```python
from build123d import *

# Parameters (mm, degrees)
SKETCH_2_W               = 20
SKETCH_2_H               = 30
EXTRUDE_1_DEPTH          = 60
SKETCH_3_W               = 18
SKETCH_3_H               = 28
CUT_EXTRUDE_1_DEPTH      = 61
CUT_EXTRUDE_1_DEPTH_BACK = 61
SKETCH_5_W               = 20
SKETCH_5_H               = 14
CUT_EXTRUDE_3_DEPTH      = 1
CUT_EXTRUDE_3_DEPTH_BACK = 31
SKETCH_6_R               = 2.025
CUT_EXTRUDE_4_DEPTH      = 31
SKETCH_7_R               = 2.025
CUT_EXTRUDE_5_DEPTH      = 1
CUT_EXTRUDE_5_DEPTH_BACK = 31


with BuildPart() as part:
    # 草图2 → 凸台-拉伸1 (new body, symmetric)
    with BuildSketch(Plane(origin=(0, 0, 0), x_dir=(1, 0, 0), z_dir=(0, 1, 0))):
        Rectangle(SKETCH_2_W, SKETCH_2_H)
    extrude(amount=EXTRUDE_1_DEPTH, both=True)

    # 草图3 → 切除-拉伸1 (cut, two sides)
    with BuildSketch(Plane(origin=(0, 0, 0), x_dir=(1, 0, 0), z_dir=(0, 1, 0))) as cut_extrude_1_sk:
        Rectangle(SKETCH_3_W, SKETCH_3_H)
    extrude(amount=CUT_EXTRUDE_1_DEPTH, mode=Mode.SUBTRACT)
    extrude(cut_extrude_1_sk.sketch, amount=-CUT_EXTRUDE_1_DEPTH_BACK, mode=Mode.SUBTRACT)

    # 草图5 → 切除-拉伸3 (cut, two sides)
    with BuildSketch(Plane.XY.offset(15)) as cut_extrude_3_sk:
        with Locations((0, -53)):
            Rectangle(SKETCH_5_W, SKETCH_5_H)
    extrude(amount=CUT_EXTRUDE_3_DEPTH, mode=Mode.SUBTRACT)
    extrude(cut_extrude_3_sk.sketch, amount=-CUT_EXTRUDE_3_DEPTH_BACK, mode=Mode.SUBTRACT)

    # 草图6 → 切除-拉伸4 (cut, through all)
    with BuildSketch(Plane.XY.offset(15)):
        with Locations((0, -33.5)):
            Circle(SKETCH_6_R)
    extrude(amount=-CUT_EXTRUDE_4_DEPTH, mode=Mode.SUBTRACT)

    # 草图7 → 切除-拉伸5 (cut, two sides)
    with BuildSketch(Plane.XY.offset(15)) as cut_extrude_5_sk:
        with Locations((0, 50)):
            Circle(SKETCH_7_R)
        with Locations((0, 30)):
            Circle(SKETCH_7_R)
        with Locations((0, 10)):
            Circle(SKETCH_7_R)
    extrude(amount=CUT_EXTRUDE_5_DEPTH, mode=Mode.SUBTRACT)
    extrude(cut_extrude_5_sk.sketch, amount=-CUT_EXTRUDE_5_DEPTH_BACK, mode=Mode.SUBTRACT)


solid = part.part
```
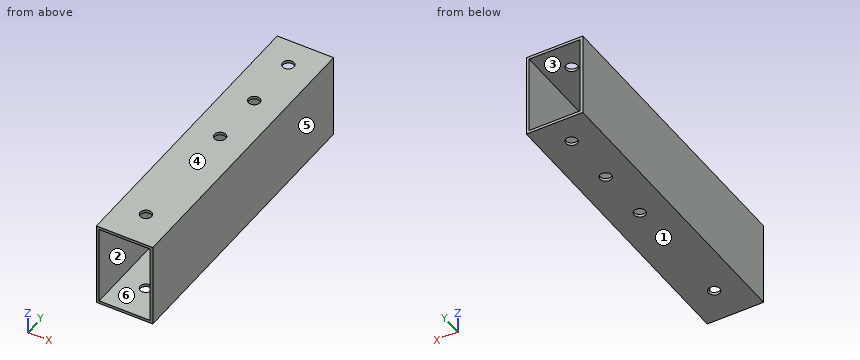
Input: part model. Units: mm. Frame: model coordinates. Face numbers are marked on the shaded views. A direction names the side the tool comes from. Give positions to 0.01 mm unless a question says otherwise; leave off trailing zeros. Order: outer loops, then holes, each group sorted by start corner. A loop starts at its lowest first (then second) coordinate and runs counter-clockwise, first axis right, second up. Notation, with made-up numbers: M -36,17.5 L 15,17.5 A21 ccw 15,33.5 Z; hole C -22,-6 d10. An arc over 180 degrees is marked long. Return JSON: item names as keys, results as strings.
Item 1: Ray query, probe 1 along Y at (x, z) = (0, -14.25) (3 decimals); probe 2 along Z at (x, y) = (-5.25, 18); probe 3 along X at (y, z) = (-36, -4.25). Return the intervals inside material, ascending.
Solutions:
{"probe 1": "-46 to -35.525, -31.475 to 7.975, 12.025 to 27.975, 32.025 to 47.975, 52.025 to 60", "probe 2": "-15 to -14, 14 to 15", "probe 3": "-10 to -9, 9 to 10"}
Item 2: Cut plane A-A (y = 47). Return loops of the section in (x, z).
Solutions:
{"outline": "M -10,-15 L 10,-15 L 10,15 L -10,15 Z; hole M -9,-14 L 9,-14 L 9,14 L -9,14 Z"}
Item 3: Pull-direction query (X, two-part tool) for the marked faces 3, 4, 5 and 6; classes: +X half, -X half, draft (parallel to the pull), parting line (faces both ways), or undercut.
Solutions:
{"face 3": "undercut", "face 4": "draft", "face 5": "+X half", "face 6": "undercut"}
Item 4: Cut plane C-C (z = -7). Return loops of the section in (x, y), then the cut area to 3 significant figures.
Solutions:
{"outline": "M -10,-46 L -9,-46 L -9,60 L -10,60 Z; M 9,-46 L 10,-46 L 10,60 L 9,60 Z", "area": "212 mm^2"}
Item 5: Cut plane B-B (x = 5.25). Return loops of the section in (y, z).
Solutions:
{"outline": "M -46,-15 L 60,-15 L 60,-14 L -46,-14 Z; M -46,14 L 60,14 L 60,15 L -46,15 Z"}
Item 6: Cut plane D-D (y = -33.5). Return loops of the section in (x, z) (3 decimals).
Solutions:
{"outline": "M -10,-15 L -2.025,-15 L -2.025,-14 L -9,-14 L -9,14 L -2.025,14 L -2.025,15 L -10,15 Z; M 2.025,-15 L 10,-15 L 10,15 L 2.025,15 L 2.025,14 L 9,14 L 9,-14 L 2.025,-14 Z"}
Item 7: Access query for the marked faces 1 and 2. Directions: +Z, -Z, +X, -X, +Y, -Y. A direction counts if a zero-diameter tool reaches every point of the face in a straight line with its end or side. Return the directions, or none.
Solutions:
{"face 1": "-Z, +X, -X, +Y, -Y", "face 2": "+Y, -Y"}
Item 8: First-contact query: P1, Ø3, axis at x = 0, y = 50, coming from the -Z side. Flat tip, straight axial feed; report the tip coordinate or a pass-through.
Solutions:
{"P1": "through"}
